```python
from build123d import *

# Parameters (mm, degrees)
F0_W     = 63.5
F0_H     = 69.85
F0_W_2   = 50.8
F0_H_2   = 57.15
F1_DEPTH = 6.35
F2_R     = 1.27
F3_DEPTH = 63.501
F4_R     = 3.175
F5_R     = 1.27
F6_DEPTH = 63.501


with BuildPart() as f1:
    # F0 (on Front) → F1 (new body)
    with BuildSketch(Plane.XZ):
        with Locations((31.75, -34.925)):
            Rectangle(F0_W, F0_H)
        with Locations((31.75, -34.925)):
            Rectangle(F0_W_2, F0_H_2, mode=Mode.SUBTRACT)
    extrude(amount=-F1_DEPTH)

    # F2 (on face) → F3 (cut, through all)
    with BuildSketch(Plane(origin=(0, 0, 0), x_dir=(0, -1, 0), z_dir=(-1, 0, 0))):
        with Locations((-3.175, -66.675)):
            Circle(F2_R)
    extrude(amount=-F3_DEPTH, mode=Mode.SUBTRACT)

    # F4
    f4_edges = [f1.edges().sort_by_distance(p)[0] for p in [
        (31.75, 6.35, -69.85),
    ]]
    fillet(f4_edges, radius=F4_R)

    # F5 (on face) → F6 (cut, through all)
    with BuildSketch(Plane.YZ.offset(63.5)):
        with Locations((3.175, -12.7)):
            Circle(F5_R)
    extrude(amount=-F6_DEPTH, mode=Mode.SUBTRACT)


solid = f1.part
```
Can you work these out from the model? Positions are in its coordinate system, mm. A direction names the side the tool comes from. Round coordinates to 2 decimals unless told otherwise and drop trailing zeros. Loops run counter-clockwise (first coordinate to the right, second up) from the corner with the lowest first, then second, coordinate; pieces in that order, holes last. Notation, with made-up numbers: (-26, -19.5) -> (9, -19.5) arc R21 cw to (9, -6.5) -> close; hole circle Ø9 at (-15.75, 69.5). An arc over 180 degrees is marked (long way). One line per item, written item: value. Start each with the question number.
1. If we mould it in two halves opening along Z, with no side actions, what happens to faces 1 (the cylindrical face through (3.22, 2.9, -13.94)), 2 (the flat face through (60, 0, -34)), 3 (the cylindrical face through (32.19, 5.4, -68.94))? For each: pulls with the +Z half, pulls with the -Z half, needs draft (parallel to the pull), parting line crosses it, or undercut.
2. For pin 1 (2 mm diameter, centred on x = 12.5, y = 5, fed in from -Z), with a flat end and sliding along its axis, tell me the tip position at first contact or that it passes through.
3. If we section it at D-D, the plane y = 1: Write out the boundary of the cut face in (x, z), then the cut area to 3 significant figures.
4. For faces 4 (the flat face through (63.5, 3, -35)), 5 (the flat face through (57.15, 3, -35)), which set-ups out of +Z, -Z, +X, -X, +Y, -Y let a thin tool reach every point of the face, with its end or its side?
5. If we section it at C-C, the plane z = -26: Write out the boundary of the cut face in (x, y), then the cut area to 3 significant figures.
6. If we section it at B-B, the plane z = -12.7: Write out the boundary of the cut face in (x, y) (3 decimals).
7. If we section it at A-A, the plane x = 20: Write out the boundary of the cut face in (y, z) (3 decimals).
8. If I drill on probe 1 along X at (y, z) = (4.25, -41.5); probe 2 along Z at (x, y) = (45, 1); probe 3 along Z at (x, y) = (17, 2.25), over which ranges is the centre line in solid material (lowest first)?
Calculated:
1. face 1: undercut
1. face 2: needs draft
1. face 3: pulls with the -Z half
2. pin 1: stops at z = -69.74
3. outline: (0, -69.85) -> (63.5, -69.85) -> (63.5, 0) -> (0, 0) -> close; hole (6.35, -63.5) -> (57.15, -63.5) -> (57.15, -6.35) -> (6.35, -6.35) -> close
3. area: 1,530 mm²
4. face 4: +Z, -Z, +X, +Y, -Y
4. face 5: +Y, -Y
5. outline: (0, 0) -> (6.35, 0) -> (6.35, 6.35) -> (0, 6.35) -> close; (57.15, 0) -> (63.5, 0) -> (63.5, 6.35) -> (57.15, 6.35) -> close
5. area: 80.6 mm²
6. outline: (0, 0) -> (6.35, 0) -> (6.35, 1.905) -> (0, 1.905) -> close; (0, 4.445) -> (6.35, 4.445) -> (6.35, 6.35) -> (0, 6.35) -> close; (57.15, 0) -> (63.5, 0) -> (63.5, 1.905) -> (57.15, 1.905) -> close; (57.15, 4.445) -> (63.5, 4.445) -> (63.5, 6.35) -> (57.15, 6.35) -> close
7. outline: (0, -69.85) -> (3.175, -69.85) arc R3.175 ccw to (6.35, -66.675) -> (6.35, -63.5) -> (0, -63.5) -> close; (0, -6.35) -> (6.35, -6.35) -> (6.35, 0) -> (0, 0) -> close; hole circle Ø2.54 at (3.175, -66.675)
8. probe 1: x = 0 to 6.35, 57.15 to 63.5
8. probe 2: z = -69.85 to -63.5, -6.35 to 0
8. probe 3: z = -69.85 to -67.55, -65.8 to -63.5, -6.35 to 0
